Model file for the job. Use its own axes, mm. A direction names the side the tool comes from. Give positions to 0.01 mm unless a question says otherwise; leave off trailing zeros. Loops run counter-clockwise (first coordinate to the right, second up) from the corner with the lowest first, then second, coordinate; pieces in that order, holes last. Notation, with made-up numbers: (-29.75, 40) - (24.25, 40) arc R26 ccw to (24.25, 62) - close; hole circle Ø5 at (82, 80). An arc over 180 degrees is marked (long way). Use a Markdown table: item, result.
from build123d import *

# Parameters (mm, degrees)
BOSS_EXTRUDE1_DEPTH = 10
SKETCH4_R           = 2
CUT_EXTRUDE1_DEPTH  = 10
CUT_EXTRUDE2_START  = -10
CUT_EXTRUDE2_DEPTH  = 10
SKETCH4_5_R         = 12.5
CUT_EXTRUDE3_DEPTH  = 10
CUT_EXTRUDE4_START  = -10
CUT_EXTRUDE4_DEPTH  = 10
SKETCH5_W           = 5
SKETCH5_H           = 15
BOSS_EXTRUDE2_DEPTH = 10
SKETCH7_W           = 5
SKETCH7_H           = 15
BOSS_EXTRUDE4_DEPTH = 12


with BuildPart() as part:
    # Sketch2 → Boss-Extrude1 (new body)
    # profile 1 of 2: a face of its own
    with BuildSketch(Plane.XY):
        Polygon((-25.980762114, 60.470053838), (-31.754264805, 60.470053838), (-60.893163975, 10), (-60.893163975, 0), (-60.893163975, -52.735026919), (-60.893163975, -57.735026919), (60.893163975, -57.735026919), (60.893163975, -52.735026919), (60.893163975, 0), (60.893163975, 10), (31.754264805, 60.470053838), (25.980762114, 60.470053838), align=None)
        with BuildLine():
            Line((-54.893163975, 10.392304845), (-29.707782181, 54.014665721))
            Line((-29.707782181, 54.014665721), (-3, 54.014665721))
            Line((-3, 54.014665721), (-3, 24.819347292))
            ThreePointArc((-3, 24.819347292), (0, 25), (3, 24.819347292))
            Line((3, 24.819347292), (3, 54.014665721))
            Line((3, 54.014665721), (29.707782181, 54.014665721))
            Line((29.707782181, 54.014665721), (54.893163975, 10.392304845))
            Line((54.893163975, 10.392304845), (54.893163975, -28.228481382))
            Line((54.893163975, -28.228481382), (22.99418526, -9.811597435))
            ThreePointArc((22.99418526, -9.811597435), (21.650635095, -12.5), (19.99418526, -15.007749857))
            Line((19.99418526, -15.007749857), (54.893163975, -35.156684613))
            Line((54.893163975, -35.156684613), (54.893163975, -52.735026919))
            Line((54.893163975, -52.735026919), (-54.893163975, -52.735026919))
            Line((-54.893163975, -52.735026919), (-54.893163975, -35.156684613))
            Line((-54.893163975, -35.156684613), (-19.99418526, -15.007749857))
            ThreePointArc((-19.99418526, -15.007749857), (-21.650635095, -12.5), (-22.99418526, -9.811597435))
            Line((-22.99418526, -9.811597435), (-54.893163975, -28.228481382))
            Line((-54.893163975, -28.228481382), (-54.893163975, 10.392304845))
        make_face(mode=Mode.SUBTRACT)
    # profile 2 of 2: a face of its own
    with BuildSketch(Plane.XY):
        with BuildLine():
            ThreePointArc((3, 24.819347292), (0, 25), (-3, 24.819347292))
            ThreePointArc((-3, 24.819347292), (-21.650635095, 12.5), (-22.99418526, -9.811597435))
            ThreePointArc((-22.99418526, -9.811597435), (-21.650635095, -12.5), (-19.99418526, -15.007749857))
            ThreePointArc((-19.99418526, -15.007749857), (0, -25), (19.99418526, -15.007749857))
            ThreePointArc((19.99418526, -15.007749857), (21.650635095, -12.5), (22.99418526, -9.811597435))
            ThreePointArc((22.99418526, -9.811597435), (24.493413722, -5.007263149), (25, 0))
            Line((25, 0), (24.879996994, 2.446579159))
            ThreePointArc((24.879996994, 2.446579159), (17.873408924, 17.479738368), (3, 24.819347292))
        make_face()
    extrude(amount=BOSS_EXTRUDE1_DEPTH)

    # Sketch4 → Cut-Extrude1 (cut)
    with BuildSketch(Plane.XY.offset(10)):
        with BuildLine():
            ThreePointArc((-13.026091256, 10.923412772), (-10.861247602, 10.541065364), (-9.653063206, 12.377645895))
            ThreePointArc((-9.653063206, 12.377645895), (-9.773085515, 13.06005624), (-10.118747085, 13.66056212))
            ThreePointArc((-10.118747085, 13.66056212), (-11.653063206, 12.377645895), (-13.026091256, 10.923412772))
        make_face()
        with BuildLine():
            ThreePointArc((-13.026091256, 10.923412772), (-11.653063206, 12.377645895), (-10.118747085, 13.66056212))
            ThreePointArc((-10.118747085, 13.66056212), (-13.024011819, 13.83383953), (-13.026091256, 10.923412772))
        make_face()
        with Locations((12.377645895, 11.653063206)):
            Circle(SKETCH4_R)
        with Locations((11.653063206, -12.377645895)):
            Circle(SKETCH4_R)
        with Locations((-12.377645895, -11.653063206)):
            Circle(SKETCH4_R)
    extrude(amount=-CUT_EXTRUDE1_DEPTH, mode=Mode.SUBTRACT)

    # Sketch4_4 → Cut-Extrude2 (cut)
    with BuildSketch(Plane.XY.offset(10).offset(CUT_EXTRUDE2_START)):
        with BuildLine():
            Line((-13.106268079, 21.289099019), (-3, 21.289099019))
            Line((-3, 21.289099019), (-3, 24.819347292))
            ThreePointArc((-3, 24.819347292), (-8.244309011, 23.601512005), (-13.106268079, 21.289099019))
        make_face()
        with BuildLine():
            Line((3, 24.819347292), (3, 21.289099019))
            Line((3, 21.289099019), (13.106268079, 21.289099019))
            ThreePointArc((13.106268079, 21.289099019), (8.244309011, 23.601512005), (3, 24.819347292))
        make_face()
        with BuildLine():
            Line((-18.989077055, -7.037341973), (-18.989077055, 16.260841079))
            ThreePointArc((-18.989077055, 16.260841079), (-24.443440144, 5.245782491), (-23.989077055, -7.037341973))
            Line((-23.989077055, -7.037341973), (-18.989077055, -7.037341973))
        make_face()
        with BuildLine():
            ThreePointArc((24.879996994, 2.446579159), (22.996355637, 9.806509441), (18.989077055, 16.260841079))
            Line((18.989077055, 16.260841079), (18.989077055, -7.037341973))
            Line((18.989077055, -7.037341973), (23.989077055, -7.037341973))
            ThreePointArc((23.989077055, -7.037341973), (24.745978728, -3.554790685), (25, 0))
            Line((25, 0), (24.879996994, 2.446579159))
        make_face()
        with BuildLine():
            Line((15.832343221, -19.347788198), (-15.832343221, -19.347788198))
            ThreePointArc((-15.832343221, -19.347788198), (0, -25), (15.832343221, -19.347788198))
        make_face()
    extrude(amount=CUT_EXTRUDE2_DEPTH, mode=Mode.SUBTRACT)

    # Sketch4_5 → Cut-Extrude3 (cut)
    with BuildSketch(Plane.XY.offset(10)):
        Circle(SKETCH4_5_R)
    extrude(amount=-CUT_EXTRUDE3_DEPTH, mode=Mode.SUBTRACT)

    # Sketch4_6 → Cut-Extrude4 (cut)
    with BuildSketch(Plane.XY.offset(10).offset(CUT_EXTRUDE4_START)):
        with BuildLine():
            Line((-22.99418526, -9.811597435), (-18.989077055, -7.037341973))
            Line((-18.989077055, -7.037341973), (-23.989077055, -7.037341973))
            ThreePointArc((-23.989077055, -7.037341973), (-23.532548901, -8.439143452), (-22.99418526, -9.811597435))
        make_face()
        with BuildLine():
            Line((23.989077055, -7.037341973), (18.989077055, -7.037341973))
            Line((18.989077055, -7.037341973), (22.99418526, -9.811597435))
            ThreePointArc((22.99418526, -9.811597435), (23.532548901, -8.439143452), (23.989077055, -7.037341973))
        make_face()
    extrude(amount=CUT_EXTRUDE4_DEPTH, mode=Mode.SUBTRACT)

    # Sketch5 → Boss-Extrude2 (add)
    with BuildSketch(Plane(origin=(-54.893163975, 0, 0), x_dir=(0, 0, -1), z_dir=(1, 0, 0))):
        with Locations((-7.5, -45.235026919)):
            Rectangle(SKETCH5_W, SKETCH5_H)
    extrude(amount=BOSS_EXTRUDE2_DEPTH)

    # Sketch7 → Boss-Extrude4 (add)
    with BuildSketch(Plane.ZY.offset(-54.893163975)):
        with Locations((7.5, -45.235026919)):
            Rectangle(SKETCH7_W, SKETCH7_H)
    extrude(amount=BOSS_EXTRUDE4_DEPTH)


solid = part.part
(1) Slice it at A-A, the plane x = 0. Write the cut outline in (y, z).
Computed:
| item | result |
|---|---|
| outline | (-57.74, 0) - (-52.74, 0) - (-52.74, 10) - (-57.74, 10) - close; (-19.35, 0) - (-12.5, 0) - (-12.5, 10) - (-19.35, 10) - close; (12.5, 0) - (60.47, 0) - (60.47, 10) - (12.5, 10) - close |
(2) Slice it at B-B, the plane y = -44. Write the cut outline in (x, z), plus the area to 3 significant figures.
Computed:
| item | result |
|---|---|
| outline | (-60.89, 0) - (-54.89, 0) - (-54.89, 5) - (-44.89, 5) - (-44.89, 10) - (-60.89, 10) - close; (42.89, 5) - (54.89, 5) - (54.89, 0) - (60.89, 0) - (60.89, 10) - (42.89, 10) - close |
| area | 230 mm² |
(3) Drill centre lines: probe 1 along Y at (x, z) = (0, 3.25); probe 2 along Y at (x, z) = (4, 1.25); probe 3 along X at (y, z) = (27.5, 7.25). Where is each one in solid material? Low to high. Write a range as [from, to].
Computed:
| item | result |
|---|---|
| probe 1 | [-57.74, -52.74], [-19.35, -12.5], [12.5, 60.47] |
| probe 2 | [-57.74, -52.74], [-19.35, -11.84], [11.84, 21.29], [54.01, 60.47] |
| probe 3 | [-50.79, -45.02], [-3, 3], [45.02, 50.79] |
(4) 3-axis set-ups, long thin cutter, end or side, ignore diameter. For faces 1 (the flat face through (60.893, -24, 5)), 2 (the flat face through (54.893, -44, 3)), 3 (the flat face through (54.893, -9, 5)): which of +Z, -Z, +X, -X, +Y, -Y reach the whole face in a straight line?
Computed:
| item | result |
|---|---|
| face 1 | +Z, -Z, +X, +Y, -Y |
| face 2 | -Z |
| face 3 | +Z, -Z |
(5) Mould opens along Y. For faces 4 (the flat face through (-50, -45, 5)), 5 (the flat face through (-1, -57.735, 5)), 6 (the flat face through (-46.12, 35.59, 4.93)) say: pulls with the +Y half, pulls with the -Y half, needs draft (parallel to the pull), parting line crosses it, or undercut.
Computed:
| item | result |
|---|---|
| face 4 | undercut |
| face 5 | pulls with the -Y half |
| face 6 | pulls with the +Y half |
(6) Slice it at D-D, the plane y = 41. Write the cut outline in (x, z).
Computed:
| item | result |
|---|---|
| outline | (-43, 0) - (-37.22, 0) - (-37.22, 10) - (-43, 10) - close; (-3, 0) - (3, 0) - (3, 10) - (-3, 10) - close; (37.22, 0) - (43, 0) - (43, 10) - (37.22, 10) - close |
(7) Pin check, flat tips, straight feed: P1, Ø3, axis at x = -12.38, y = -11.65, coming from the +Z side; P2, Ø3.5, axis at x = 49.5, y = -42, coming from the -Z side; P3, Ø1.5, axis at x = 45.5, z = 3, coming from the +Y side; P4, Ø1.5, axis at x = 51, z = 8, coming from the +Y side. Stop position of each tip, or through.
Computed:
| item | result |
|---|---|
| P1 | through |
| P2 | z = 5 |
| P3 | y = 37.96 |
| P4 | y = 28.43 |
(8) Slice it at C-C, the plane y = 0. Write the cut outline in (x, z).
Computed:
| item | result |
|---|---|
| outline | (-60.89, 0) - (-54.89, 0) - (-54.89, 10) - (-60.89, 10) - close; (-18.99, 0) - (-12.5, 0) - (-12.5, 10) - (-18.99, 10) - close; (12.5, 0) - (18.99, 0) - (18.99, 10) - (12.5, 10) - close; (54.89, 0) - (60.89, 0) - (60.89, 10) - (54.89, 10) - close |
